Can you work these out from the model? Positions are in its coordinate system, mm. Face numbers are marked on the shaded views. A direction names the side the tool comes from. Round coordinates to 2 decimals unless told otherwise and drop trailing zeros. Loops run counter-clockwise (first coordinate to the right, second up) from the corner with the lowest first, then second, coordinate; pieces in that order, holes last. Notation, with made-up numbers: M 57.25,72.25 L 73.25,72.25 A8 cw 73.25,85.25 Z; hole C 55,56.5 d7. An arc over 180 degrees is marked long. Use a Markdown table: item, result. Add a question column.
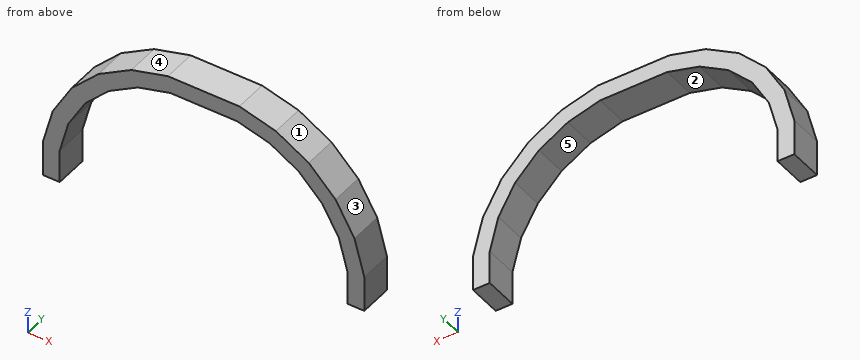
```python
from build123d import *

# Parameters (mm, degrees)
F1_DEPTH = 10


with BuildPart() as f1:
    # F0 (on Front) → F1 (new body)
    with BuildSketch(Plane.XZ):
        Polygon((0, 0), (5.000002, 0), (5.000002, 10), (7.588192, 19.659258), (12.588192, 28.319512), (19.65926, 35.39058), (28.319514, 40.39058), (37.978773, 42.978771), (47.978773, 42.978771), (47.978773, 47.978773), (37.32051, 47.978773), (26.389586, 45.04984), (16.589187, 39.391577), (8.587195, 31.389586), (2.928932, 21.589187), (0, 10.658263), align=None)
    extrude(amount=F1_DEPTH)

    # F2: F1 across face


with BuildPart() as f1_1:
    add(f1.part)
    add(f1.part.mirror(Plane(origin=(47.978773, -5, 45.478772), x_dir=(0, 1, 0), z_dir=(1, 0, 0))))


solid = f1_1.part
```
(1) I'm going to push flat-ended pins straight in: pin 1 (5 mm diameter, centred on x = 55, y = -9, fed in from -Z); pin 2 (1.5 mm diameter, centred on y = -2, z = 33, fed in from +X); pin 3 (4 mm diameter, centred on x = 31.5, y = -7.5, fed in from +Z). Where does each tip first touch, or does it pass through?
(2) Suppose I cut it at D-D on z = 18. List the corners of the cut face in (x, y) for me.
(3) If I drill on probe 1 along X at (y, z) = (-7.25, 7); probe 2 along Z at (x, y) = (39, -2.75); probe 3 along X at (y, z) = (-7.5, 20.5), over which ranges is the centre line in solid material (lowest first)? Write a range as [from, to].
(4) Suppose I cut it at C-C on x = 53. List the corners of the cut face in (y, z) for me, and give its area (3 significant figures).
(5) On a 3-axis mill with a long thin cutter (end or side, diameter ignored), from which of +Z, -Z, +X, -X, +Y, -Y can I reach the whole of each face in a straight line? I mean the marked faces 1 and 2. Say none if no direction works.
(6) Thinking about a two-plate mould opening in X: for the marked faces 3, 4 and 5, which applies, released by +X, released by -X, zero draft, split by the parting line, or undercut?
(7) Suppose I cut it at B-B on z = 33. List the corners of the cut face in (x, y) for me.
(8) Suppose I cut it at A-A on y = -4. List the corners of the cut face in (x, z) for me, and give its area (3 significant figures).
Results below:
| question | item | result |
|---|---|---|
| 1 | pin 1 | stops at z = 42.98 |
| 1 | pin 2 | stops at x = 86.51 |
| 1 | pin 3 | stops at z = 46.96 |
| 2 | outline | M 1.97,-10 L 7.14,-10 L 7.14,0 L 1.97,0 Z; M 88.81,-10 L 93.99,-10 L 93.99,0 L 88.81,0 Z |
| 3 | probe 1 | x = [0, 5], [90.96, 95.96] |
| 3 | probe 2 | z = [42.98, 47.98] |
| 3 | probe 3 | x = [2.64, 8.07], [87.88, 93.32] |
| 4 | outline | M -10,42.98 L 0,42.98 L 0,47.98 L -10,47.98 Z |
| 4 | area | 50.0 mm² |
| 5 | face 1 | +Z, +X, +Y, -Y |
| 5 | face 2 | -Z, +Y, -Y |
| 6 | face 3 | released by +X |
| 6 | face 4 | released by -X |
| 6 | face 5 | undercut |
| 7 | outline | M 10.2,-10 L 17.27,-10 L 17.27,0 L 10.2,0 Z; M 78.69,-10 L 85.76,-10 L 85.76,0 L 78.69,0 Z |
| 8 | outline | M 0,0 L 5,0 L 5,10 L 7.59,19.66 L 12.59,28.32 L 19.66,35.39 L 28.32,40.39 L 37.98,42.98 L 57.98,42.98 L 67.64,40.39 L 76.3,35.39 L 83.37,28.32 L 88.37,19.66 L 90.96,10 L 90.96,0 L 95.96,0 L 95.96,10.66 L 93.03,21.59 L 87.37,31.39 L 79.37,39.39 L 69.57,45.05 L 58.64,47.98 L 37.32,47.98 L 26.39,45.05 L 16.59,39.39 L 8.59,31.39 L 2.93,21.59 L 0,10.66 Z |
| 8 | area | 739 mm² |
